Answer from the drawing. Dimensions are ordinates in mm from the lowest x, y and z of the part. A direction names the side the tool comes from. Give positions to 0.01 mm unless a question says otherwise; leave off trailing zeros. Order: outer loops, then holes, each group sorted by start corner. A loop starts at its lowest first (then second) coordinate and runs counter-clockwise, first axis right, second up. Notation, with made-up numbers: M 75,14 L 118,14 A21 ccw 118,30 Z; hole C 43.5,67 d7. An arc over 180 degrees is marked long. One line per item, written item: value.
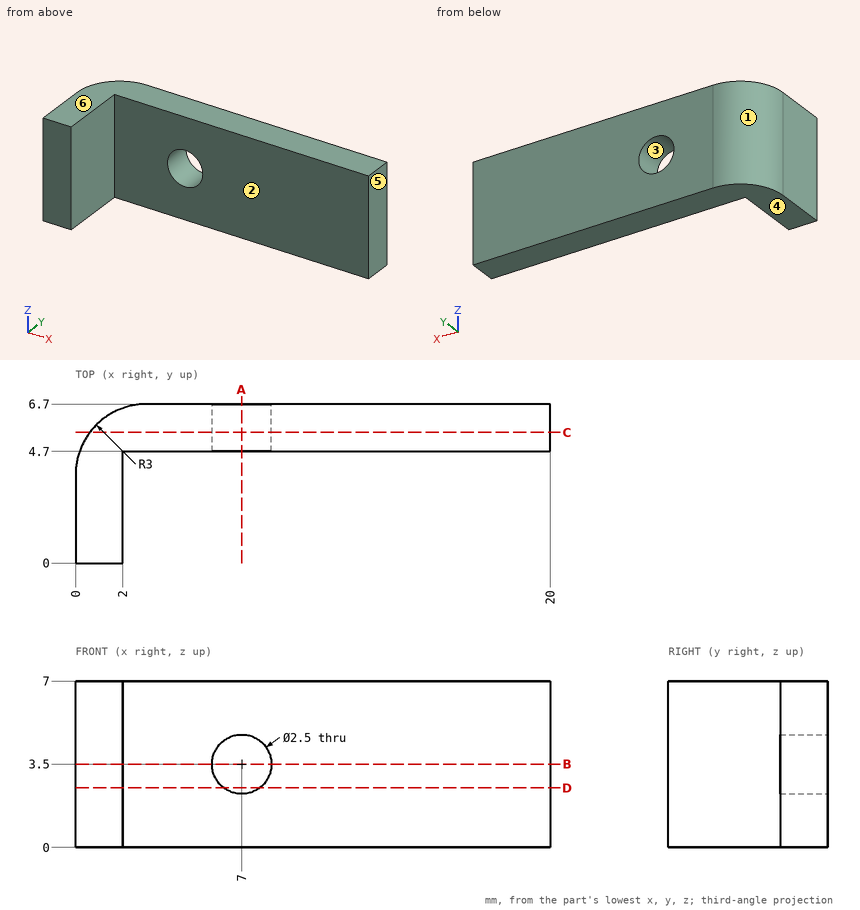
(1) Determine the mould class of the marked faces 3, 4, 5 and 6 for opening direction Z: pulls with the +Z half, pulls with the -Z half, needs draft (parallel to the pull), parting line crosses it, or undercut.
Findings:
face 3: undercut
face 4: pulls with the -Z half
face 5: needs draft
face 6: pulls with the +Z half
(2) Section C-C, the plane y = 5.5 is taken. Give the vertices of the cut face in (x, z), then the cut area to 3 significant figures.
Findings:
outline: M 0.6,0 L 20,0 L 20,7 L 0.6,7 Z; hole C 7,3.5 d2.5
area: 131 mm^2
(3) Find the intervals of material crossed by probe 1 along Z at (x, y) = (7, 5.3); probe 2 along Y at (x, z) = (3.25, 0.75); probe 3 along X at (y, z) = (4.75, 3.75), in increasing order. Write a range as from..to.
Findings:
probe 1: z = 0..2.25, 4.75..7
probe 2: y = 4.7..6.7
probe 3: x = 0.19..5.78, 8.22..20
(4) Which of the six approach directions +Z, -Z, +X, -X, +Y, -Y give full straight-line access (tool end or side, diameter ignored) to the marked faces 1 and 2?
Findings:
face 1: +Z, -Z, -X, +Y
face 2: +Z, -Z, +X, -Y
(5) Given P1, Ø3, axis at x = 7, z = 3.5, coming from the -Y side, flat-ended and moving along its own axis, determine where the tip first touches the part or whether it passes through.
Findings:
P1: stops at y = 4.7
(6) Section D-D, the plane z = 2.5 is taken. Give the vertices of the cut face in (x, y), then the cut area to 3 significant figures.
Findings:
outline: M 0,0 L 2,0 L 2,4.7 L 6.25,4.7 L 6.25,6.7 L 3,6.7 A3 ccw 0,3.7 Z; M 7.75,4.7 L 20,4.7 L 20,6.7 L 7.75,6.7 Z
area: 44.5 mm^2
(7) Section B-B, the plane z = 3.5 is taken. Give the vertices of the cut face in (x, y), then the cut area to 3 significant figures.
Findings:
outline: M 0,0 L 2,0 L 2,4.7 L 5.75,4.7 L 5.75,6.7 L 3,6.7 A3 ccw 0,3.7 Z; M 8.25,4.7 L 20,4.7 L 20,6.7 L 8.25,6.7 Z
area: 42.5 mm^2
(8) Section A-A, the plane x = 7 is taken. Give the vertices of the cut face in (y, z), then the cut area to 3 significant figures.
Findings:
outline: M 4.7,0 L 6.7,0 L 6.7,2.25 L 4.7,2.25 Z; M 4.7,4.75 L 6.7,4.75 L 6.7,7 L 4.7,7 Z
area: 9.00 mm^2
